For this review, use the dimensioned drawing (mm, ordinates from the lowest corner) and the shaded views. A direction names the side the tool comes from. Round coordinates to 2 decimals unless told otherwise and drop trailing zeros. Loops run counter-clockwise (first coordinate to the right, second up) from the corner with the lowest first, then second, coordinate; pieces in that order, holes last. Notation, with made-up numbers: (49.25, -27) -> (62.25, -27) arc R11 cw to (62.25, -7) -> close; hole circle Ø2 at (-36, 70.25). An arc over 180 degrees is marked (long way). Use one line per item in the form item = value. Start each with the question number.
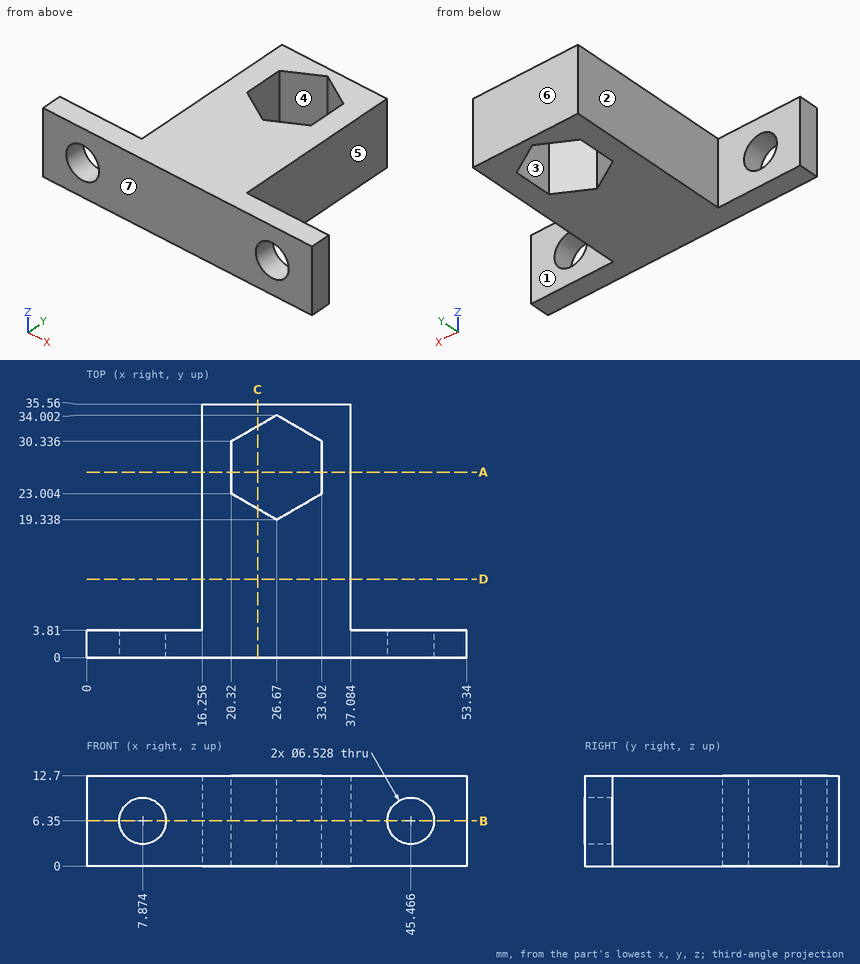
Item 1: Wall thickness on line 1 (X direction, y = 1.9, z = 6.35); line 2 (X direction, y = 2, z = 3.75) (1 decimal); line 3 (X direction, y = 26, z = 3.5): over which ranges is each line inside the solid? List them lowest first.
Item 2: Draft analysis for pull direction Y (two halves, no side actions). For the marked faces 4, 5, 6 and 7, state which applies: +Y half, -Y half, draft (parallel to the pull), parting line (faces both ways), or undercut.
Item 3: Take a section at C-C on x = 24. Give the boundary of the cut face in (y, z).
Item 4: Take a section at A-A on y = 26. Give the boundary of the cut face in (x, z), plus the area to 3 significant figures.
Item 5: For P1, Ø1.5, axis at y = 14, z = 9, coming from the +X side; P2, Ø7.5, axis at x = 45.466, z = 6.35, coming from the -Y side; P3, Ø4, axis at y = 15, z = 8, coming from the -X side, all flat-tipped, find the tip position at first contact; note any pin that passes through.
Item 6: Take a section at B-B on z = 6.35. Give the boundary of the cut face in (x, y), plus the area to 3 significant figures.
Item 7: Take a section at D-D on y = 11. Give the boundary of the cut face in (x, z).
Item 8: Machinability: for the marked faces 1, 2 and 3, which of the approach directions +Z, -Z, +X, -X, +Y, -Y give a long, thin tool a straight path to every point of the face, cutting with its end or side? Answer none if there is none.
Results:
q1.line_1 = 0 to 4.61, 11.14 to 42.2, 48.73 to 53.34
q1.line_2 = 0 to 5.9, 9.8 to 43.5, 47.4 to 53.3
q1.line_3 = 16.26 to 20.32, 33.02 to 37.08
q2.face_4 = undercut
q2.face_5 = draft
q2.face_6 = +Y half
q2.face_7 = -Y half
q3.outline = (0, 0) -> (20.88, 0) -> (20.88, 12.7) -> (0, 12.7) -> close; (32.46, 0) -> (35.56, 0) -> (35.56, 12.7) -> (32.46, 12.7) -> close
q4.outline = (16.26, 0) -> (20.32, 0) -> (20.32, 12.7) -> (16.26, 12.7) -> close; (33.02, 0) -> (37.08, 0) -> (37.08, 12.7) -> (33.02, 12.7) -> close
q4.area = 103 mm2
q5.P1 = 37.08
q5.P2 = 0
q5.P3 = 16.26
q6.outline = (0, 0) -> (4.61, 0) -> (4.61, 3.81) -> (0, 3.81) -> close; (11.14, 0) -> (42.2, 0) -> (42.2, 3.81) -> (37.08, 3.81) -> (37.08, 35.56) -> (16.26, 35.56) -> (16.26, 3.81) -> (11.14, 3.81) -> close; (48.73, 0) -> (53.34, 0) -> (53.34, 3.81) -> (48.73, 3.81) -> close; hole (20.32, 23) -> (26.67, 19.34) -> (33.02, 23) -> (33.02, 30.34) -> (26.67, 34) -> (20.32, 30.34) -> close
q6.area = 675 mm2
q7.outline = (16.26, 0) -> (37.08, 0) -> (37.08, 12.7) -> (16.26, 12.7) -> close
q8.face_1 = +Z, -Z, +X, +Y
q8.face_2 = +Z, -Z, -X, +Y
q8.face_3 = +Z, -Z
